Could you check a few things on this model? Use its own coordinates, in mm. A direction names the side the tool comes from. Give positions to 0.01 mm unless a question says otherwise; leave off trailing zeros. Write each loop counter-clockwise with the first axis right and the second up, starting at its lowest first coordinate (ties: lowest second). Pieces come first, ordered by that corner, then holes. Notation, with made-up numbers: M -36,7 L 21,7 A19 cw 21,22 Z; hole C 6.25,18 d5. An arc over 180 degrees is marked long. Use one line per item in the form item = value.
from build123d import *

# Parameters (mm, degrees)
CROQUIS1_R              = 2
SALIENTE_EXTRUIR1_DEPTH = 2.5
SALIENTE_EXTRUIR2_START = -2.5
SALIENTE_EXTRUIR2_DEPTH = 2.5
SALIENTE_EXTRUIR3_START = -2.5
SALIENTE_EXTRUIR3_DEPTH = 2.5
CROQUIS3_R              = 1.5
CORTAR_EXTRUIR1_DEPTH   = 10


# Read off the part's stored shape, not the designer's step: Saliente-Extruir2
with BuildPart() as part:
    # Croquis1 → Saliente-Extruir1 (new body)
    # profile 1 of 5: a face of its own
    with BuildSketch(Plane.XY):
        with BuildLine():
            Line((-21.120737491, -7.779592428), (-4.410977671, -7.779592428))
            ThreePointArc((-4.410977671, -7.779592428), (-3.91525524, -8.214329332), (-4.281568148, -8.762555341))
            Line((-4.281568148, -8.762555341), (-20.42195671, -13.087359421))
            ThreePointArc((-20.42195671, -13.087359421), (-18.774789479, -20.700029026), (-16.394943343, -28.116377909))
            Line((-16.394943343, -28.116377909), (-0.254554781, -23.791573829))
            ThreePointArc((-0.254554781, -23.791573829), (0.336794507, -24.083195026), (0.124854741, -24.707549444))
            Line((0.124854741, -24.707549444), (-14.346221754, -33.062429354))
            ThreePointArc((-14.346221754, -33.062429354), (-10.27145788, -40.865753752), (-5.363777272, -48.173984957))
            ThreePointArc((-5.363777272, -48.173984957), (-4.165388027, -48.929294708), (-2.76728992, -48.70136646))
            Line((-2.76728992, -48.70136646), (19.509218146, -35.840018532))
            ThreePointArc((19.509218146, -35.840018532), (20.480258523, -34.447083978), (20.030579853, -32.809715608))
            ThreePointArc((20.030579853, -32.809715608), (7.934326683, 0), (20.030579853, 32.809715608))
            ThreePointArc((20.030579853, 32.809715608), (20.480258523, 34.447083978), (19.509218146, 35.840018532))
            Line((19.509218146, 35.840018532), (-2.76728992, 48.70136646))
            ThreePointArc((-2.76728992, 48.70136646), (-4.165388027, 48.929294708), (-5.363777272, 48.173984957))
            ThreePointArc((-5.363777272, 48.173984957), (-10.27145788, 40.865753752), (-14.346221754, 33.062429354))
            Line((-14.346221754, 33.062429354), (0.124854741, 24.707549444))
            ThreePointArc((0.124854741, 24.707549444), (0.336794507, 24.083195026), (-0.254554781, 23.791573829))
            Line((-0.254554781, 23.791573829), (-16.394943343, 28.116377909))
            ThreePointArc((-16.394943343, 28.116377909), (-18.774789479, 20.700029026), (-20.42195671, 13.087359421))
            Line((-20.42195671, 13.087359421), (-4.281568148, 8.762555341))
            ThreePointArc((-4.281568148, 8.762555341), (-3.91525524, 8.214329332), (-4.410977671, 7.779592428))
            Line((-4.410977671, 7.779592428), (-21.120737491, 7.779592428))
            ThreePointArc((-21.120737491, 7.779592428), (-21.5, 0), (-21.120737491, -7.779592428))
        make_face()
        with Locations((-8.186800297, -38.489385282)):
            Circle(CROQUIS1_R, mode=Mode.SUBTRACT)
        with Locations((-15.877012, -19.92357189)):
            Circle(CROQUIS1_R, mode=Mode.SUBTRACT)
        with Locations((-5.251827911, -17.076562394)):
            Circle(CROQUIS1_R, mode=Mode.SUBTRACT)
        with Locations((1.339479145, -32.989385282)):
            Circle(CROQUIS1_R, mode=Mode.SUBTRACT)
        with Locations((-18.5, 0)):
            Circle(CROQUIS1_R, mode=Mode.SUBTRACT)
        with Locations((-15.877012, 19.92357189)):
            Circle(CROQUIS1_R, mode=Mode.SUBTRACT)
        with Locations((-7.5, 0)):
            Circle(CROQUIS1_R, mode=Mode.SUBTRACT)
        with Locations((-5.251827911, 17.076562394)):
            Circle(CROQUIS1_R, mode=Mode.SUBTRACT)
        with Locations((-8.186800297, 38.489385282)):
            Circle(CROQUIS1_R, mode=Mode.SUBTRACT)
        with Locations((1.339479145, 32.989385282)):
            Circle(CROQUIS1_R, mode=Mode.SUBTRACT)
    # profile 2 of 5: a face of its own
    with BuildSketch(Plane.XY):
        with BuildLine():
            ThreePointArc((-14.346221754, 33.062429354), (-15.411978596, 30.606550436), (-16.394943343, 28.116377909))
            Line((-16.394943343, 28.116377909), (-0.254554781, 23.791573829))
            ThreePointArc((-0.254554781, 23.791573829), (0.336794507, 24.083195026), (0.124854741, 24.707549444))
            Line((0.124854741, 24.707549444), (-14.346221754, 33.062429354))
        make_face()
    # profile 3 of 5: a face of its own
    with BuildSketch(Plane.XY):
        with BuildLine():
            ThreePointArc((-20.42195671, 13.087359421), (-20.815770531, 10.43932438), (-21.120737491, 7.779592428))
            Line((-21.120737491, 7.779592428), (-4.410977671, 7.779592428))
            ThreePointArc((-4.410977671, 7.779592428), (-3.91525524, 8.214329332), (-4.281568148, 8.762555341))
            Line((-4.281568148, 8.762555341), (-20.42195671, 13.087359421))
        make_face()
    # profile 4 of 5: a face of its own
    with BuildSketch(Plane.XY):
        with BuildLine():
            ThreePointArc((-4.281568148, -8.762555341), (-3.91525524, -8.214329332), (-4.410977671, -7.779592428))
            Line((-4.410977671, -7.779592428), (-21.120737491, -7.779592428))
            ThreePointArc((-21.120737491, -7.779592428), (-20.815770531, -10.43932438), (-20.42195671, -13.087359421))
            Line((-20.42195671, -13.087359421), (-4.281568148, -8.762555341))
        make_face()
    # profile 5 of 5: a face of its own
    with BuildSketch(Plane.XY):
        with BuildLine():
            Line((-0.254554781, -23.791573829), (-16.394943343, -28.116377909))
            ThreePointArc((-16.394943343, -28.116377909), (-15.411978596, -30.606550436), (-14.346221754, -33.062429354))
            Line((-14.346221754, -33.062429354), (0.124854741, -24.707549444))
            ThreePointArc((0.124854741, -24.707549444), (0.336794507, -24.083195026), (-0.254554781, -23.791573829))
        make_face()
    extrude(amount=SALIENTE_EXTRUIR1_DEPTH)

    # Saliente-Extruir2 outline → Saliente-Extruir2 (add)
    with BuildSketch(Plane.XY.offset(SALIENTE_EXTRUIR2_START)):
        with BuildLine():
            Line((-0.254554781, -23.791573829), (-16.394943343, -28.116377909))
            ThreePointArc((-16.394943343, -28.116377909), (-15.411978595, -30.606550436), (-14.346221754, -33.062429354))
            Line((-14.346221754, -33.062429354), (0.124854741, -24.707549444))
            ThreePointArc((0.124854741, -24.707549444), (0.336794507, -24.083195026), (-0.254554781, -23.791573829))
        make_face()
        with BuildLine():
            Line((-4.410977671, -7.779592428), (-21.120737491, -7.779592428))
            ThreePointArc((-21.120737491, -7.779592428), (-20.815770531, -10.43932438), (-20.42195671, -13.087359421))
            Line((-20.42195671, -13.087359421), (-4.281568148, -8.762555341))
            ThreePointArc((-4.281568148, -8.762555341), (-3.91525524, -8.214329332), (-4.410977671, -7.779592428))
        make_face()
        with BuildLine():
            Line((-4.281568148, 8.762555341), (-20.42195671, 13.087359421))
            ThreePointArc((-20.42195671, 13.087359421), (-20.815770531, 10.43932438), (-21.120737491, 7.779592428))
            Line((-21.120737491, 7.779592428), (-4.410977671, 7.779592428))
            ThreePointArc((-4.410977671, 7.779592428), (-3.91525524, 8.214329332), (-4.281568148, 8.762555341))
        make_face()
        with BuildLine():
            Line((-16.394943343, 28.116377909), (-0.254554781, 23.791573829))
            ThreePointArc((-0.254554781, 23.791573829), (0.336794507, 24.083195026), (0.124854741, 24.707549444))
            Line((0.124854741, 24.707549444), (-14.346221754, 33.062429354))
            ThreePointArc((-14.346221754, 33.062429354), (-15.411978595, 30.606550436), (-16.394943343, 28.116377909))
        make_face()
    extrude(amount=SALIENTE_EXTRUIR2_DEPTH)

    # Croquis2 → Saliente-Extruir3 (add)
    with BuildSketch(Plane.XY.offset(2.5).offset(SALIENTE_EXTRUIR3_START)):
        with BuildLine():
            ThreePointArc((20.030579853, 32.809715608), (11.054709029, 17.484255625), (7.934326683, 0))
            Line((7.934326683, 0), (10.654225828, 0))
            ThreePointArc((10.654225828, 0), (10.744136996, 2.931183608), (11.013532431, 5.85134584))
            Line((11.013532431, 5.85134584), (29.845645811, 11.606363843))
            Line((29.845645811, 11.606363843), (46.670524679, 11.606363843))
            Line((46.670524679, 11.606363843), (46.670524679, 34.626841689))
            Line((46.670524679, 34.626841689), (20.50887875, 34.144811605))
            ThreePointArc((20.50887875, 34.144811605), (20.392040458, 33.433445566), (20.030579853, 32.809715608))
        make_face()
        with BuildLine():
            Line((10.654225828, 0), (7.934326683, 0))
            ThreePointArc((7.934326683, 0), (11.054709029, -17.484255625), (20.030579853, -32.809715608))
            ThreePointArc((20.030579853, -32.809715608), (20.392040458, -33.433445566), (20.50887875, -34.144811605))
            Line((20.50887875, -34.144811605), (46.670524679, -34.626841689))
            Line((46.670524679, -34.626841689), (46.670524679, -11.606363843))
            Line((46.670524679, -11.606363843), (29.845645811, -11.606363843))
            Line((29.845645811, -11.606363843), (11.013532431, -5.85134584))
            ThreePointArc((11.013532431, -5.85134584), (10.744136996, -2.931183608), (10.654225828, 0))
        make_face()
    extrude(amount=SALIENTE_EXTRUIR3_DEPTH)

    # Croquis3 → Cortar-Extruir1 (cut)
    with BuildSketch(Plane.XY.offset(2.5)):
        with Locations((35.845645811, -17.5)):
            Circle(CROQUIS3_R)
        with Locations((35.845645811, 17.5)):
            Circle(CROQUIS3_R)
    extrude(amount=-CORTAR_EXTRUIR1_DEPTH, mode=Mode.SUBTRACT)


solid = part.part
1) I want a section at C-C, the plane y = 29.5. Please give me the cut outline in (x, z).
Checked values:
outline = M -15.86,-2.5 L -8.18,-2.5 L -8.18,0 L 46.67,0 L 46.67,2.5 L -15.86,2.5 Z
2) I want a section at B-B, the plane x = 18. Please give me the cut outline in (y, z).
Checked values:
outline = M -36.71,0 L -7.99,0 L -7.99,2.5 L -36.71,2.5 Z; M 7.99,0 L 36.71,0 L 36.71,2.5 L 7.99,2.5 Z
3) For pin 1 Ø3 at (x, z) = (20, -1) entering from -Y; pin 2 Ø4.5 at (x, y) = (1.34, 32.99) entering from -Z; pin 3 Ø1.2 at (x, z) = (39, 1.5) entering from -Y, each with a flat end and sliding along its axis, tell me the tip position at first contact or that it passes through.
Checked values:
pin_1 = -36.2
pin_2 = 0
pin_3 = -34.5
4) If I drill on L1, parallel to Y at x = -11, z = -2.15; L2, parallel to Y at x = -10, z = -0.55; L3, parallel to Z at x = 5, y = 17, over which ranges is the centre line in solid material (lowest first)?
Checked values:
L1 = -31.13 to -26.67, -10.56 to -7.78, 7.78 to 10.56, 26.67 to 31.13
L2 = -30.55 to -26.4, -10.29 to -7.78, 7.78 to 10.29, 26.4 to 30.55
L3 = 0 to 2.5
5) For faces 4 (the flat face through (38, 11.606, 1)), 5 (the cylindrical face through (-4.185, -48.925, 1.232)), 6 (the flat face through (-8.212, -25.924, -1.268)), 7 (the flat face through (-13, -7.78, -1)), which set-ups out of +Z, -Z, +X, -X, +Y, -Y let a thin tool reach every point of the face, with its end or its side?
Checked values:
face_4 = +Z, -Z, +X
face_5 = +Z, -Z, -Y
face_6 = -Z, -X
face_7 = -Z, +X, -X
6) Thinking about a two-plate mould opening in Y: for faces 1 (the flat face through (-15, -10, -2.5)), 2 (the flat face through (20.3, 8.69, 1.23)), 3 (the flat face through (8.22, -42.36, 1.23)), which applies, released by +Y, released by -Y, zero draft, split by the parting line, or undercut?
Checked values:
face_1 = zero draft
face_2 = undercut
face_3 = released by -Y
7) I want a section at A-A, the plane z = -1.35. Please give me the cut outline in (x, y), plus the area to 3 significant figures.
Checked values:
outline = M -21.12,-7.78 A79.98 ccw -20.42,-13.09 L -4.28,-8.76 A0.5 ccw -4.41,-7.78 Z; M -21.12,7.78 L -4.41,7.78 A0.5 ccw -4.28,8.76 L -20.42,13.09 A79.98 ccw Z; M -16.39,-28.12 A79.98 ccw -14.35,-33.06 L 0.12,-24.71 A0.5 ccw -0.25,-23.79 Z; M -16.39,28.12 L -0.25,23.79 A0.5 ccw 0.12,24.71 L -14.35,33.06 A79.98 ccw Z
area = 212 mm2
